```python
from build123d import *

# Parameters (mm, degrees)
SKETCH1_R           = 1.714400001
SKETCH1_R_2         = 3.4289
SKETCH1_R_3         = 3.2384
SKETCH1_R_4         = 1.7144
BOSS_EXTRUDE1_DEPTH = 2.54
CHAMFER1_SIZE       = 1.27


with BuildPart() as part:
    # Sketch1 → Boss-Extrude1 (new body)
    with BuildSketch(Plane(origin=(0, 0, 0), x_dir=(0, 0, -1), z_dir=(1, 0, 0))):
        with BuildLine():
            Line((62.3394, 9.4286), (9.441, 9.4286))
            add(Edge.make_bspline(
                [(9.441, 9.4286), (6.94, 9.427), (4.5283, 8.4336), (2.7592, 6.6645)],
                knots=[0.3, 0.3, 0.3, 0.3, 0.4, 0.4, 0.4, 0.4], degree=3))
            add(Edge.make_bspline(
                [(2.7592, 6.6645), (0.9915, 4.897), (-0.0016, 2.4997), (0, 0)],
                knots=[0.4, 0.4, 0.4, 0.4, 0.5, 0.5, 0.5, 0.5], degree=3))
            add(Edge.make_bspline(
                [(0, 0), (0.0015, -2.5473), (0.9866, -5.2522), (2.7684, -7.0749)],
                knots=[0.5, 0.5, 0.5, 0.5, 0.6, 0.6, 0.6, 0.6], degree=3))
            add(Edge.make_bspline(
                [(2.7684, -7.0749), (4.5268, -8.8738), (6.923, -9.9024), (9.441, -9.9008)],
                knots=[0.6, 0.6, 0.6, 0.6, 0.7, 0.7, 0.7, 0.7], degree=3))
            Line((9.441, -9.9008), (62.3394, -9.9008))
            add(Edge.make_bspline(
                [(62.3394, -9.9008), (64.857, -9.8992), (67.2635, -8.868), (69.0205, -7.066)],
                knots=[0.8, 0.8, 0.8, 0.8, 0.9, 0.9, 0.9, 0.9], degree=3))
            add(Edge.make_bspline(
                [(69.0205, -7.066), (70.8008, -5.2404), (71.782, -2.547), (71.7804, -0.0002)],
                knots=[0.9, 0.9, 0.9, 0.9, 1, 1, 1, 1], degree=3))
            add(Edge.make_bspline(
                [(71.7804, -0.0002), (71.7789, 2.4992), (70.7829, 4.9074), (69.0128, 6.6729)],
                knots=[0, 0, 0, 0, 0.1, 0.1, 0.1, 0.1], degree=3))
            add(Edge.make_bspline(
                [(69.0128, 6.6729), (67.2418, 8.4394), (64.8408, 9.4302), (62.3394, 9.4286)],
                knots=[0.1, 0.1, 0.1, 0.1, 0.2, 0.2, 0.2, 0.2], degree=3))
        make_face()
        with Locations((3.6195, 0.005300001)):
            Circle(SKETCH1_R, mode=Mode.SUBTRACT)
        with Locations((13.5437, 2.4303)):
            Circle(SKETCH1_R_2, mode=Mode.SUBTRACT)
        with Locations((28.5051, 0.2713)):
            Circle(SKETCH1_R_3, mode=Mode.SUBTRACT)
        with Locations((41.3701, 0.2713)):
            Circle(SKETCH1_R_3, mode=Mode.SUBTRACT)
        with Locations((54.0701, 0.2713)):
            Circle(SKETCH1_R_3, mode=Mode.SUBTRACT)
        with Locations((68.1608, 0.0053)):
            Circle(SKETCH1_R_4, mode=Mode.SUBTRACT)
    extrude(amount=BOSS_EXTRUDE1_DEPTH)

    # Chamfer1
    chamfer1_edges = [part.edges().sort_by_distance(p)[0] for p in [
        (2.54, 0.005300001, -1.905099999),
        (2.54, 0.0053, -66.4464),
    ]]
    chamfer(chamfer1_edges, length=CHAMFER1_SIZE)


solid = part.part
```
Model file for the job. Use its own axes, mm. Coordinates: 2 decimals unless noted, no trailing zeros. Order: outer loops, then holes, each group sorted by start corner. A loop starts at its lowest first (then second) coordinate and runs counter-clockwise, first axis right, second up. Notation, with made-up numbers: (4.25, 39) -> (49.25, 39) arc R34 ccw to (49.25, 75) -> close; hole circle Ø6 at (-22, -14). An arc over 180 degrees is marked (long way). Answer as a JSON object with one key per item and string values. Group by question number.
1) Pull direction Z, two halves, no side cores. Call faces 1 (the face through (1, 9.429, -36)), 2 (the face through (0.63, 0.08, -66.45)): +Z half, -Z half, draft (parallel to the pull), parting line (faces both ways), or undercut.
2) Cut at A-A, the plane z = -29. Write the cut outline in (x, y).
3) Drill centre lines: L1, parallel to Z at x = 0.2, y = -1.75; L2, parallel to Y at x = 1.7, z = -12; L3, parallel to Y at x = 1.8, z = -13. Where is each one in solid material? Low to high.
4) Cut at B-B, the plane x = 0.8. Count the separate pieces of the cut face and the enclosed holes in it, then the cut area to 3 significant figures.
5) Flat gauge pins, fed straight in: pin 1 (4 mm diameter, centred on y = 0.01, z = -3.62, fed in from +X); pin 2 (6 mm diameter, centred on y = 2.43, z = -13.54, fed in from +X). Where does each tip first touch, or does it go through?
Check values:
{
 "1": {"face 1": "draft", "face 2": "undercut"},
 "2": {"outline": "(0, -9.9) -> (2.54, -9.9) -> (2.54, -2.93) -> (0, -2.93) -> close; (0, 3.47) -> (2.54, 3.47) -> (2.54, 9.43) -> (0, 9.43) -> close"},
 "3": {"L1": "z = -71.63 to -56.6, -51.54 to -43.9, -38.84 to -31.04, -25.97 to -0.15", "L2": "y = -9.9 to -0.63, 5.49 to 9.43", "L3": "y = -9.9 to -0.96, 5.82 to 9.43"},
 "4": {"separate pieces": "1", "enclosed holes": "6", "area": "1,160 mm²"},
 "5": {"pin 1": "stops at x = 1.56", "pin 2": "passes through"}
}
